Geometry check sheet. Reference: the model listing, model coordinates, mm. A direction names the side the tool comes from. Coordinates: 2 decimals unless noted, no trailing zeros. Write each loop counter-clockwise with the first axis right and the second up, starting at its lowest first coordinate (ties: lowest second). Pieces come first, ordered by that corner, then holes. Notation, with made-up numbers: (68, 69) -> (118, 69) arc R31 ccw to (118, 97) -> close; hole circle Ø9 at (88, 26). An arc over 180 degrees is marked (long way). One line per question, with ' | ' between items.
from build123d import *

# Parameters (mm, degrees)
F0_W     = 0.5
F0_H     = 15
F2_R     = 0.5
F3_DEPTH = 1
F4_R     = 0.4
F5_DEPTH = 0.3


with BuildPart() as f1:
    # F0 (on Front) → F1 (revolve)
    with BuildSketch(Plane.XZ):
        with Locations((0.25, 7.5)):
            Rectangle(F0_W, F0_H)
    revolve(axis=Axis((0, 0, 7.5), (0, 0, 1)))

    # F2 (on face) → F3 (join)
    with BuildSketch(Plane.XY.offset(15)):
        Polygon((0.75, 0.0006401425), (0.3744456203, 0.6498391241), (-0.3755543797, 0.6491989816), (-0.75, -0.0006401425), (-0.3744456203, -0.6498391241), (0.3755543797, -0.6491989816), align=None)
        Circle(F2_R, mode=Mode.SUBTRACT)
        Circle(F2_R)
    extrude(amount=F3_DEPTH)

    # F4 (on face) → F5 (cut)
    with BuildSketch(Plane.XY.offset(16)):
        Circle(F4_R)
    extrude(amount=-F5_DEPTH, mode=Mode.SUBTRACT)


solid = f1.part
1. Cross-section at C-C on z = 5. Record the boundary of the cut face in (x, y), and give its area (3 significant figures).
Worked answers:
outline: circle Ø1 at (0, 0) | area: 0.785 mm²
2. Cross-section at A-A on y = -0.15. Record the boundary of the cut face in (x, z), and give its area (3 significant figures).
Worked answers:
outline: (-0.66, 15) -> (-0.48, 15) -> (-0.48, 0) -> (0.48, 0) -> (0.48, 15) -> (0.66, 15) -> (0.66, 16) -> (0.37, 16) -> (0.37, 15.7) -> (-0.37, 15.7) -> (-0.37, 16) -> (-0.66, 16) -> close | area: 15.4 mm²
3. Cross-section at B-B on x = 0. Record the boundary of the cut face in (y, z).
Worked answers:
outline: (-0.65, 15) -> (-0.5, 15) -> (-0.5, 0) -> (0.5, 0) -> (0.5, 15) -> (0.65, 15) -> (0.65, 16) -> (0.4, 16) -> (0.4, 15.7) -> (-0.4, 15.7) -> (-0.4, 16) -> (-0.65, 16) -> close
4. Material ranges on line 1 (Y direction, x = 0, z = 15.95); line 2 (Z direction, x = 0.2, y = -0.55); line 3 (Y direction, x = -0.05, z = 11.25), recorded low to high. Write a range as from..to.
Worked answers:
line 1: -0.65..-0.4, 0.4..0.65 | line 2: 15..16 | line 3: -0.5..0.5
5. Tool access check on faces 1 (the face through (0, 0, 0)), 2 (the face through (-0.108, -0.488, 7.605)). Record the directions out of +Z, -Z, +X, -X, +Y, -Y that give a thin tool (end or side, any length) a straight path to the whole face; none if there is none.
Worked answers:
face 1: -Z, +X, -X, +Y, -Y | face 2: -Z
